Source: CAD feature listing. Evaluate the final solid. Frame: model axes, mm. A direction names the side the tool comes from. Round coordinates to 2 decimals unless told otherwise and drop trailing zeros. Order: outer loops, then holes, each group sorted by start corner. A loop starts at its lowest first (then second) coordinate and runs counter-clockwise, first axis right, second up. Notation, with made-up numbers: M -36,3.25 L -25,3.25 A21 cw -25,42.25 Z; hole C -5,80.25 d2. An arc over 180 degrees is marked long. Use CSV: the item, a comma, the result in double quotes. Start each with the question number.
```python
from build123d import *

# Parameters (mm, degrees)
SKETCH1_R           = 3.5
SKETCH1_R_2         = 6
SKETCH1_R_3         = 2.5
SKETCH1_R_4         = 1.5
SKETCH1_R_5         = 10.5
BOSS_EXTRUDE1_DEPTH = 10
FILLET1_R           = 10
FILLET2_R           = 10
FILLET3_R           = 10
FILLET4_R           = 10


with BuildPart() as part:
    # Sketch1 → Boss-Extrude1 (new body)
    with BuildSketch(Plane(origin=(0, 0, 0), x_dir=(1, 0, 0), z_dir=(0, 1, 0))):
        with BuildLine():
            Line((76.000002703, -25), (76.000002703, -35))
            Line((76.000002703, -35), (126.000002703, -35))
            Line((126.000002703, -35), (126.000002703, 35))
            Line((126.000002703, 35), (76.000002703, 35))
            Line((76.000002703, 35), (76.000002703, 25))
            Line((76.000002703, 25), (0, 25))
            ThreePointArc((0, 25), (-25, 0), (0, -25))
            Line((0, -25), (76.000002703, -25))
        make_face()
        with Locations(Location((101.000002703, 24, 0), (0, 0, 270))):
            Circle(SKETCH1_R, mode=Mode.SUBTRACT)
        with Locations(Location((101.000002703, -24, 0), (0, 0, 270))):
            Circle(SKETCH1_R, mode=Mode.SUBTRACT)
        with Locations(Location((101.000002703, 0, 0), (0, 0, 270))):
            Circle(SKETCH1_R_2, mode=Mode.SUBTRACT)
        with Locations(Location((35, 0, 0), (0, 0, 270))):
            Circle(SKETCH1_R_3, mode=Mode.SUBTRACT)
        with Locations(Location((0, 15, 0), (0, 0, 270))):
            Circle(SKETCH1_R_4, mode=Mode.SUBTRACT)
        with Locations(Location((12.990377534, -7.499997966, 0), (0, 0, 270))):
            Circle(SKETCH1_R_4, mode=Mode.SUBTRACT)
        with Locations(Location((-12.990376356, -7.500008143, 0), (0, 0, 270))):
            Circle(SKETCH1_R_4, mode=Mode.SUBTRACT)
        with Locations(Location((0, 0, 0), (0, 0, 270))):
            Circle(SKETCH1_R_5, mode=Mode.SUBTRACT)
    extrude(amount=BOSS_EXTRUDE1_DEPTH)

    # Fillet1
    fillet1_edges = [part.edges().sort_by_distance(p)[0] for p in [
        (126.000002703, 5, 35),
    ]]
    fillet(fillet1_edges, radius=FILLET1_R)

    # Fillet2
    fillet2_edges = [part.edges().sort_by_distance(p)[0] for p in [
        (76.000002703, 5, 35),
    ]]
    fillet(fillet2_edges, radius=FILLET2_R - 0.0001)  # a hair under: the kernel refuses the full size

    # Fillet3
    fillet3_edges = [part.edges().sort_by_distance(p)[0] for p in [
        (76.000002703, 5, -35),
    ]]
    fillet(fillet3_edges, radius=FILLET3_R - 0.0001)  # a hair under: the kernel refuses the full size

    # Fillet4
    fillet4_edges = [part.edges().sort_by_distance(p)[0] for p in [
        (126.000002703, 5, -35),
    ]]
    fillet(fillet4_edges, radius=FILLET4_R)


solid = part.part
```
(1) Line query: line 1 along X through (y, z) = (3.75, 0); line 2 along X through (y, z) = (1.25, 7); line 3 along Z through (x, y) = (98.5, 9.25). Output: solid intervals per line, ascending.
(2) Section A-A on z = -15. Return loops of the section in (x, y).
(3) Reachability of faces 5 (the face through (-24.994, 4.93, -0.55)), 6 (the face through (37, 5, 25)), 7 (the face through (39, 5, -25)) from +Z, -Z, +X, -X, +Y, -Y: full face, straight path, thin tool, end or side. Return the list, or none.
(4) Contact query for a flat-ended pin moving along its axis: P1, Ø4, axis at y = 8, z = 12, coming from the -X side. Output: stop coordinate, or through.
(5) Draft query along X for faces 1 (the face through (95.143, 4.93, -1.301)), 2 (the face through (101, 5, 35)), 3 (the face through (97.583, 4.93, 23.241)), 4 (the face through (126, 5, 0)). Return one class per face: pulls with the +X half, pulls with the -X half, needs draft (parallel to the pull), parting line crosses it, or undercut.
(6) Section B-B on x = 35. Return loops of the section in (y, z).
(7) Section C-C on z = 0. Return loops of the section in (x, y), plus the area to 3 significant figures.
(8) Section D-D on y = 1.5. Give the number of separate pieces and of enclosed holes in the cut face, plus the area to 3 significant figures.
Results below:
1,line 1,"x = -25 to -10.5, 10.5 to 32.5, 37.5 to 95, 107 to 126"
1,line 2,"x = -24 to -14.4, -11.58 to -7.83, 7.83 to 11.58, 14.4 to 126"
1,line 3,"z = -35 to -26.45, -21.55 to -5.45, 5.45 to 21.55, 26.45 to 35"
2,outline,"M -20,0 L -1.5,0 L -1.5,10 L -20,10 Z; M 1.5,0 L 126,0 L 126,10 L 1.5,10 Z"
3,face 5,"-X, +Y, -Y"
3,face 6,"+Z, -X, +Y, -Y"
3,face 7,"-Z, -X, +Y, -Y"
4,P1,"stops at x = -22.91"
5,face 1,"undercut"
5,face 2,"needs draft"
5,face 3,"undercut"
5,face 4,"pulls with the +X half"
6,outline,"M 0,-25 L 10,-25 L 10,-2.5 L 0,-2.5 Z; M 0,2.5 L 10,2.5 L 10,25 L 0,25 Z"
7,outline,"M -25,0 L -10.5,0 L -10.5,10 L -25,10 Z; M 10.5,0 L 32.5,0 L 32.5,10 L 10.5,10 Z; M 37.5,0 L 95,0 L 95,10 L 37.5,10 Z; M 107,0 L 126,0 L 126,10 L 107,10 Z"
7,area,"1,130 mm2"
8,separate pieces,"1"
8,enclosed holes,"8"
8,area,"7,620 mm2"
